```python
from build123d import *

# Parameters (mm, degrees)
SKETCH1_W           = 12.7
SKETCH1_H           = 101.6
BOSS_EXTRUDE1_DEPTH = 6.35
SKETCH2_W           = 12.7
SKETCH2_H           = 6.35
SKETCH2_R           = 1.651
BOSS_EXTRUDE2_DEPTH = 6.35
SKETCH3_R           = 3.175
CUT_EXTRUDE1_DEPTH  = 58.851253228


with BuildPart() as part:
    # Sketch1 → Boss-Extrude1 (new body)
    with BuildSketch(Plane(origin=(0, 0, 0), x_dir=(1, 0, 0), z_dir=(0, 1, 0))):
        Rectangle(SKETCH1_W, SKETCH1_H)
    extrude(amount=BOSS_EXTRUDE1_DEPTH)

    # Sketch2 → Boss-Extrude2 (add)
    # profile 1 of 2: a face of its own
    with BuildSketch(Plane(origin=(0, 6.35, 0), x_dir=(1, 0, 0), z_dir=(0, 1, 0))):
        with Locations((0, 53.975)):
            Rectangle(SKETCH2_W, SKETCH2_H)
        with Locations(Location((0, 53.975, 0), (0, 0, 270))):
            Circle(SKETCH2_R, mode=Mode.SUBTRACT)
    # profile 2 of 2: a face of its own
    with BuildSketch(Plane(origin=(0, 6.35, 0), x_dir=(1, 0, 0), z_dir=(0, 1, 0))):
        with Locations((0, -53.975)):
            Rectangle(SKETCH2_W, SKETCH2_H)
        with Locations(Location((0, -53.975, 0), (0, 0, 270))):
            Circle(SKETCH2_R, mode=Mode.SUBTRACT)
    extrude(amount=-BOSS_EXTRUDE2_DEPTH)

    # Sketch3 → Cut-Extrude1 (cut, through all)
    with BuildSketch(Plane(origin=(0, 6.35, 0), x_dir=(1, 0, 0), z_dir=(0, 1, 0))):
        with Locations(Location((0, 38.1, 0), (0, 0, 270))):
            Circle(SKETCH3_R)
    extrude(amount=-CUT_EXTRUDE1_DEPTH, mode=Mode.SUBTRACT)


solid = part.part
```
Part model, mm, in its own coordinate system. Round coordinates to 2 decimals unless told otherwise and drop trailing zeros. Write each loop counter-clockwise with the first axis right and the second up, starting at its lowest first coordinate (ties: lowest second). Pieces come first, ordered by that corner, then holes. Notation, with made-up numbers: (-25, 72) -> (-12, 72) arc R14 cw to (-12, 89) -> close; hole circle Ø7 at (25, 36). An arc over 180 degrees is marked (long way). Return JSON: item names as keys, results as strings. Group by question number.
Q1. Saw through at B-B on z = -38.1. Write the cut outline in (x, y) (3 decimals), plus the area to 3 significant figures.
Q2. Saw through at A-A on x = 0. Write the cut outline in (y, z) (3 decimals), plus the area to 3 significant figures.
Q3. Probe L1, parallel to X at y = 4.5, z = -38.1 (3 decimals); L2, parallel to Z at x = -0.25, y = 3.5; L3, parallel to Z at x = -0.5, y = 4.75. List the from-to ranges inside material, lowest first. Write a range as [from, to].
Q4. Saw through at C-C on y = 4.5. Write the cut outline in (x, z) (3 decimals).
Q5. Mould opens along X. For faces 1 (the flat face through (0, 6.35, -1)), 2 (the flat face through (6.35, 3, 1)), 3 (the cylindrical face through (0.5, 3.22, 55.55)) say: pulls with the +X half, pulls with the -X half, needs draft (parallel to the pull), parting line crosses it, or undercut.
Answer:
{
 "1": {"outline": "(-6.35, 0) -> (-3.175, 0) -> (-3.175, 6.35) -> (-6.35, 6.35) -> close; (3.175, 0) -> (6.35, 0) -> (6.35, 6.35) -> (3.175, 6.35) -> close", "area": "40.3 mm2"},
 "2": {"outline": "(0, -57.15) -> (6.35, -57.15) -> (6.35, -55.626) -> (0, -55.626) -> close; (0, -52.324) -> (6.35, -52.324) -> (6.35, -41.275) -> (0, -41.275) -> close; (0, -34.925) -> (6.35, -34.925) -> (6.35, 52.324) -> (0, 52.324) -> close; (0, 55.626) -> (6.35, 55.626) -> (6.35, 57.15) -> (0, 57.15) -> close", "area": "644 mm2"},
 "3": {"L1": "[-6.35, -3.175], [3.175, 6.35]", "L2": "[-57.15, -55.61], [-52.34, -41.27], [-34.93, 52.34], [55.61, 57.15]", "L3": "[-57.15, -55.55], [-52.4, -41.24], [-34.96, 52.4], [55.55, 57.15]"},
 "4": {"outline": "(-6.35, -57.15) -> (6.35, -57.15) -> (6.35, 57.15) -> (-6.35, 57.15) -> close; hole circle Ø6.35 at (0, -38.1); hole circle Ø3.302 at (0, -53.975); hole circle Ø3.302 at (0, 53.975)"},
 "5": {"face 1": "needs draft", "face 2": "pulls with the +X half", "face 3": "undercut"}
}
